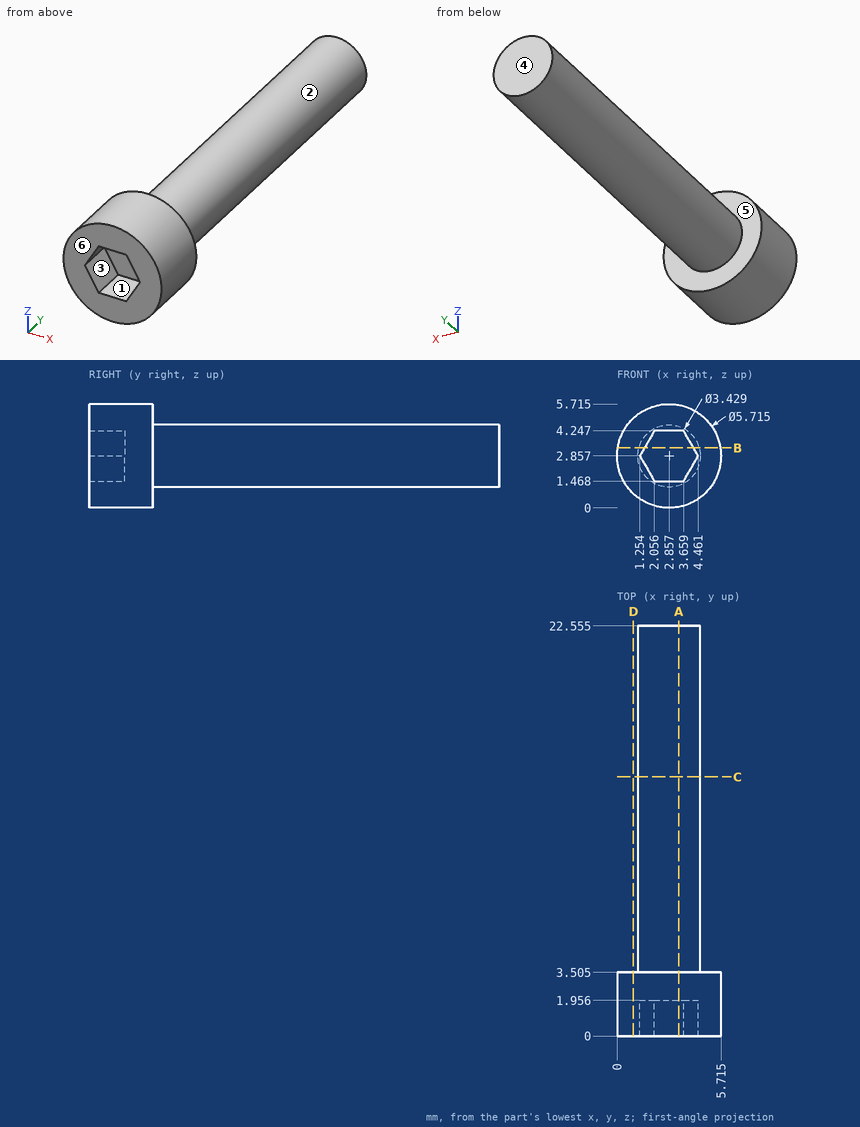
Can you work these out from the drawing? Everything is in mm from the part's minimum corner. A direction names the side the tool comes from. Give positions to 0.01 mm unless a question says otherwise; leave off trailing zeros. Write each loop counter-clockwise with the first axis right and the second up, starting at its lowest first coordinate (ties: lowest second). Pieces come first, ordered by that corner, then holes. Notation, with made-up numbers: (16, 17.25) -> (38, 17.25) arc R10 ccw to (38, 33.25) -> close; hole circle Ø4 at (-22.75, -5.5). An arc over 180 degrees is marked (long way). Write each question's results on one line, items separated by ' | '.
Item 1: Suppose I cut it at B-B on z = 3.3. Write out the boundary of the cut face in (x, y) (1 decimal).
Output:
outline: (0, 0) -> (1.5, 0) -> (1.5, 2) -> (4.2, 2) -> (4.2, 0) -> (5.7, 0) -> (5.7, 3.5) -> (4.5, 3.5) -> (4.5, 22.6) -> (1.2, 22.6) -> (1.2, 3.5) -> (0, 3.5) -> close
Item 2: Suppose I cut it at D-D on x = 0.9. Write out the boundary of the cut face in (y, z) (1 decimal), plus the area to 3 significant figures.
Output:
outline: (0, 0.8) -> (3.5, 0.8) -> (3.5, 4.9) -> (0, 4.9) -> close | area: 14.6 mm^2
Item 3: Suppose I cut it at A-A on x = 3.4. Write out the boundary of the cut face in (y, z) (1 decimal).
Output:
outline: (0, 0.1) -> (3.5, 0.1) -> (3.5, 1.2) -> (22.6, 1.2) -> (22.6, 4.5) -> (3.5, 4.5) -> (3.5, 5.7) -> (0, 5.7) -> (0, 4.2) -> (2, 4.2) -> (2, 1.5) -> (0, 1.5) -> close
Item 4: If I drill on L1, parallel to Y at x = 5.15, z = 3.7 (1 decimal); L2, parallel to Z at x = 2.95, y = 3; L3, parallel to Y at x = 4, z = 2.5 (1 decimal), over which ranges is the centre line in solid material (lowest first)?
Output:
L1: y = 0 to 3.5 | L2: z = 0 to 5.71 | L3: y = 2 to 22.6
Item 5: On a 3-axis mill with a long thin cutter (end or side, diameter ignored), from which of +Z, -Z, +X, -X, +Y, -Y can I reach the whole of each face in a straight line? I mean the marked faces 5 and 6. Say none if no direction works.
Output:
face 5: +Y | face 6: +Z, -Z, +X, -X, -Y
Item 6: Suppose I cut it at C-C on y = 14.25. Write out the boundary of the cut face in (x, z) (1 decimal).
Output:
outline: circle Ø3.4 at (2.9, 2.9)
Item 7: We'd pull the mould along Z, two halves only. Please class the marked faces 1, 2, 3 and 4: pulls with the +Z half, pulls with the -Z half, needs draft (parallel to the pull), parting line crosses it, or undercut.
Output:
face 1: undercut | face 2: parting line crosses it | face 3: undercut | face 4: needs draft
Item 8: For pin 1 Ø1.5 at (y, z) = (9.5, 1.5) entering from +X; pin 2 Ø1.5 at (y, z) = (5, 4.5) entering from +X; pin 3 Ø0.8 at (x, z) = (3, 2.5) entering from -Y, each with a flat end and sliding along its axis, tell me the tip position at first contact or that it passes through.
Output:
pin 1: stops at x = 4.46 | pin 2: stops at x = 4.32 | pin 3: stops at y = 1.96
